The drawing under review shows one solid part. Ordinate dimensions are in mm from its lowest x, y, z. A direction names the side the tool comes from. Give positions to 0.01 mm unless a question says otherwise; leave off trailing zeros. Loops run counter-clockwise (first coordinate to the right, second up) from the corner with the lowest first, then second, coordinate; pieces in that order, holes last. Notation, with made-up numbers: M 72,9 L 85,9 A19 ccw 85,18 Z; hole C 65.5,-23.75 d6. An arc over 180 degrees is marked long. One line per item, written item: value. Start each with the question number.
Q1. We need section A-A on y = 26.5. Write out the cut boundary in (x, z), plus the area to 3 significant figures.
Q2. To check wall thickness, follow line 1 along Z through (x, y) = (21, 22.5); line 2 along X through (y, z) = (13, 16); line 3 along Y through (x, z) = (13.75, 58). State the ranges of each line that lie inside material, in increasing order. Write a range as from..to.
Q3. We need section D-D on x = 28.25. Write out the cut boundary in (y, z), plus the area to 4 significant figures.
Q4. For the marked faces 1, 2 and 3, list the 3-axis set-ups (+Z, -Z, +X, -X, +Y, -Y) from which the entire face can be reached by the end or side of a thin tool; tool diameter is ignored.
Q5. We need section B-B on x = 24.25. Write out the cut boundary in (y, z).
Q6. For pin 1 (15 mm diameter, centred on x = 16.5, z = 41.5, fed in from -Y); pin 2 (9 mm diameter, centred on x = 21.5, y = 46.5, fed in from +Z), all flat-tipped, find the tip position at first contact; note any pin that passes through.
Q7. We need section C-C on z = 49.5. Write out the cut boundary in (x, y), plus the area to 3 significant figures.
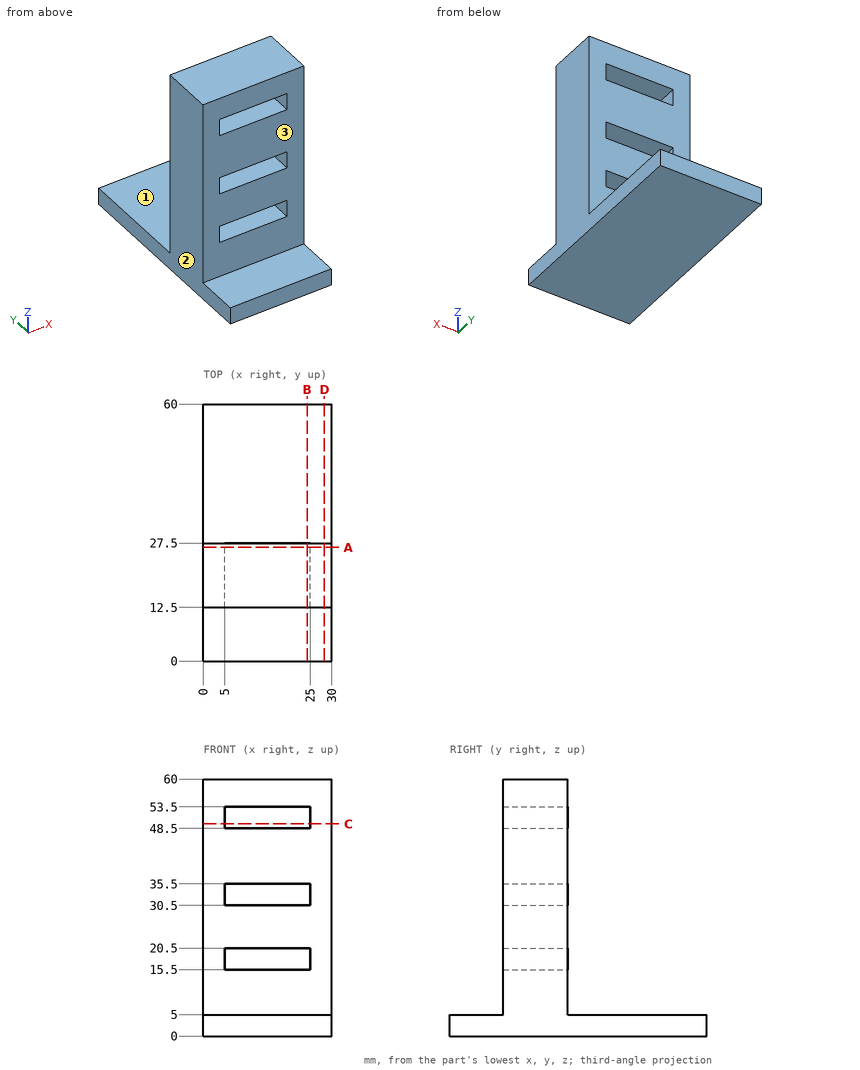
Solved:
1. outline: M 0,0 L 30,0 L 30,60 L 0,60 Z; hole M 5,15.5 L 25,15.5 L 25,20.5 L 5,20.5 Z; hole M 5,30.5 L 25,30.5 L 25,35.5 L 5,35.5 Z; hole M 5,48.5 L 25,48.5 L 25,53.5 L 5,53.5 Z
1. area: 1,500 mm2
2. line 1: 0..15.5, 20.5..30.5, 35.5..48.5, 53.5..60
2. line 2: 0..5, 25..30
2. line 3: 12.5..27.5
3. outline: M 0,0 L 60,0 L 60,5 L 27.5,5 L 27.5,60 L 12.5,60 L 12.5,5 L 0,5 Z
3. area: 1,125 mm2
4. face 1: +Z, +X, -X, +Y
4. face 2: +Z, -Z, -X, +Y, -Y
4. face 3: +Z, +X, -X, -Y
5. outline: M 0,0 L 60,0 L 60,5 L 27.5,5 L 27.5,15.5 L 12.5,15.5 L 12.5,5 L 0,5 Z; M 12.5,20.5 L 27.5,20.5 L 27.5,30.5 L 12.5,30.5 Z; M 12.5,35.5 L 27.5,35.5 L 27.5,48.5 L 12.5,48.5 Z; M 12.5,53.5 L 27.5,53.5 L 27.5,60 L 12.5,60 Z
6. pin 1: y = 12.5
6. pin 2: z = 5
7. outline: M 0,12.5 L 5,12.5 L 5,27.5 L 0,27.5 Z; M 25,12.5 L 30,12.5 L 30,27.5 L 25,27.5 Z
7. area: 150 mm2
